CAD build for the part. Positions are in the model's coordinates, mm. A direction names the side the tool comes from. Give positions to 0.01 mm unless a question says otherwise; leave off trailing zeros. Loops run counter-clockwise (first coordinate to the right, second up) from the corner with the lowest first, then second, coordinate; pieces in that order, holes last.
Autodesk Inventor part; units mm, degrees
ref_plane "SHELL Plane" through (-424.2641, -424.2641, 0) normal (0.7071, -0.7071, 0) x (0.7071, 0.7071, 0)
ref_plane "ACCESS Plane" through (-213, -1000, 0) normal (0, -1, 0) x (1, 0, 0)
ref_plane "OUTER Plane" through (-38, -800, 0) normal (0, -1, 0) x (1, 0, 0)
sketch "floor angle sketch" plane through (0, 0, 0) normal (0, 0, 1) x (1, 0, 0)
  line L0 (0, 0) -> (0, -240.1382) construction
  line L1 (0, 0) -> (0, -1000)
  line L2 (-424.2641, -424.2641) -> (424.2641, 424.2641) construction
  circle A0 centre (0, 0) radius 600 construction
  line L3 (0, 0) -> (0, -800)
  line L4 (-38, -800) -> (38, -800)
  line L5 (-213, -1000) -> (213, -1000)
  line L6 (0, 0) -> (-307.8181, -845.7234)
  line L7 (0, 0) -> (0, -700)
  line L8 (-38, -700) -> (38, -700)
  line L9 (-368.8981, -823.492) -> (-246.7381, -867.9547)
  dimension "d51" = 1200
  dimension "d52" = 45
  dimension "d54" = 0
  dimension "d55" = 0
  dimension "d56" = 426
  dimension "d58" = 76
  dimension "d59" = 76
  dimension "d60" = 0
  dimension "d61" = 700
  dimension "d62" = 130
  dimension "d63" = 20
  dimension "d64" = 800
  dimension "d65" = 900
  dimension "d66" = 1000
ref_plane "SHELL Plane" through (-424.2641, -424.2641, 0) normal (0.7071, -0.7071, 0) x (0.7071, 0.7071, 0)
ref_plane "ACCESS Plane" through (-213, -1000, 0) normal (0, -1, 0) x (1, 0, 0)
ref_plane "OUTER Plane" through (-38, -800, 0) normal (0, -1, 0) x (1, 0, 0)
ref_plane "INNER Plane" through (-38, -700, 0) normal (0, -1, 0) x (1, 0, 0)
ref_plane "CHARGE Plane" through (-368.8981, -823.492, 0) normal (-0.342, -0.9397, 0) x (0.9397, -0.342, 0)
sketch "Sketch13" plane through (-424.2641, -424.2641, 0) normal (0.7071, -0.7071, 0) x (0.7071, 0.7071, 0)
  line L0 (600, 0) -> (600, 892.6829)
  line L1 (0, 0) -> (6, 0)
  line L2 (6, 0) -> (6, 1500)
  line L3 (6, 1500) -> (0, 1500)
  line L4 (0, 1500) -> (0, 0)
  dimension "d75" = 1500
  dimension "d76" = 6
  dimension "d77" = 1200
revolve "Revolution2" add sketch "Sketch13" angle 359.9 about axis through (0, 0, 0) along (0, 0, 1)
sketch "Sketch14" plane through (-213, -1000, 0) normal (0, -1, 0) x (1, 0, 0)
  circle A0 centre (213, 960) radius 213
  line L0 (813, 1500) -> (-387, 1500)
  point P0 (213, 0)
  point P1 (-211.2641, 1500)
  point P2 (-212.0039, 1500)
  dimension "d80" = 426
  dimension "d93" = 540
extrude "ACCESS" cut sketch "Sketch14" against normal up to next
sketch "Sketch15" plane through (-38, -700, 0) normal (0, -1, 0) x (1, 0, 0)
  circle A0 centre (38, 190) radius 38
  point P0 (38, 0)
  dimension "d84" = 76
  dimension "d85" = 190
extrude "INNER" cut sketch "Sketch15" against normal up to next
sketch "Sketch16" plane through (-38, -800, 0) normal (0, -1, 0) x (1, 0, 0)
  circle A0 centre (38, 1350) radius 38
  line L0 (638, 1500) -> (-562, 1500)
  point P0 (38, 0)
  point P1 (-386.2641, 1500)
  point P2 (-387.0039, 1500)
  dimension "d89" = 76
  dimension "d92" = 150
extrude "Extrusion9" cut sketch "Sketch16" against normal up to next
equation "\"BendRadius\" = Thickness"
equation "\"BendReliefWidth\" = Thickness"
equation "\"BendReliefDepth\" = 0.5 * Thickness"
equation "\"CornerReliefSize\" = 4 * Thickness"
equation "\"MinimumRemnant\" = 2 * Thickness"
equation "\"TransitionRadius\" = BendRadius"
equation "\"JacobiRadiusSize\" = BendRadius"
equation "\"GapSize\" = Thickness"
properties part number "TZS 1202 SHELL" material "Steel"
1. Tool access for faces 4 (the face through (109.193, -584.102, 1142.882)), 5 (the face through (78.36, 588.81, 760.5)): list every direction of +Z, -Z, +X, -X, +Y, -Y with a clear straight run to the whole face (end or side of a thin tool).
Responses:
face 4: -Y
face 5: +Z, -Z
2. Probe line 1 along Y through (x, z) = (0, 336); line 2 along Y through (x, z) = (-298, 564.5); line 3 along X through (y, z) = (-81.5, 137.5). List the from-to ranges inside material, lowest first.
Responses:
line 1: y = -600 to -594, 594 to 600
line 2: y = -520.76 to -513.84, 513.84 to 520.76
line 3: x = -594.44 to -588.38, 588.38 to 594.44
3. Saw through at A-A, the plane x = 0. List the corners of the cut face in (y, z).
Responses:
outline: (-600, 0) - (-594, 0) - (-594, 152) - (-600, 152) - close; (-600, 228) - (-594, 228) - (-594, 747) - (-600, 747) - close; (-600, 1173) - (-594, 1173) - (-594, 1312) - (-600, 1312) - close; (-600, 1388) - (-594, 1388) - (-594, 1500) - (-600, 1500) - close; (594, 0) - (600, 0) - (600, 1500) - (594, 1500) - close
4. Saw through at D-D, the plane x = -140.5. List the corners of the cut face in (y, z), and give its area (3 significant figures).
Responses:
outline: (-583.32, 0) - (-577.14, 0) - (-577.14, 799.91) - (-583.32, 799.91) - close; (-583.32, 1120.09) - (-577.14, 1120.09) - (-577.14, 1500) - (-583.32, 1500) - close; (577.14, 0) - (583.32, 0) - (583.32, 1500) - (577.14, 1500) - close
area: 16,500 mm2
5. Saw through at C-C, the plane z = 793.5. List the corners of the cut face in (x, y).
Responses:
outline: (-425, -423.52) - (-420.75, -419.29) arc R594 cw (long way) to (132.84, -578.96) - (132.84, -585.11) arc R600 ccw (long way) to start; (-424.26, -424.26) arc R600 ccw to (-132.84, -585.11) - (-132.84, -578.96) arc R594 cw to (-420.02, -420.02) - close
6. Saw through at B-B, the plane y = 0. List the corners of the cut face in (x, z), and give its area (3 significant figures).
Responses:
outline: (-600, 0) - (-594, 0) - (-594, 1500) - (-600, 1500) - close; (594, 0) - (600, 0) - (600, 1500) - (594, 1500) - close
area: 18,000 mm2
7. Pull direction Z, two halves, no side cores. Call faces 1 (the face through (35.102, -596.442, 1335.446)), 2 (the face through (507, -314, 1500)), 3 (the face through (507, -314, 0)): released by +Z, released by -Z, zero draft, split by the parting line, or undercut.
Responses:
face 1: undercut
face 2: released by +Z
face 3: released by -Z
8. Drop flat-ended pins along their axis: pin 1 (2 mm diameter, centred on y = 104.5, z = 1182, fed in from +X); pin 2 (2 mm diameter, centred on y = -175, z = 386.5, fed in from +X); pin 3 (2 mm diameter, centred on y = -39, z = 1177, fed in from -X). Give the stop position or say it passes through.
Responses:
pin 1: stops at x = 591.01
pin 2: stops at x = 574.22
pin 3: stops at x = -598.8
